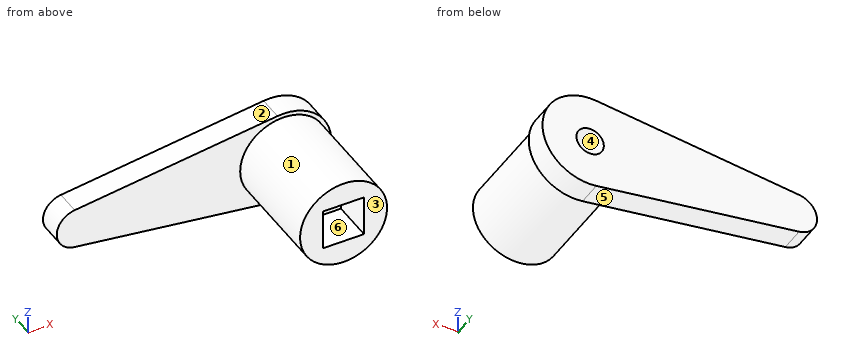
Solid Edge part; units mm, degrees
sketch "Sketch1" plane through (0, 0, 0) normal (0, 1, 0) x (-1, 0, 0)
  circle A0 centre (0, 0) radius 5.275
  circle A1 centre (0, 0) radius 1.66
extrude "Protrusion1" add sketch "Sketch1" along normal blind 8
sketch "Sketch2" plane through (0, 8, 0) normal (0, 1, 0) x (0, 0, 1)
  arc A0 (5.7252, -0.7565) -> (-5.7252, -0.7565) centre (0, 0) ccw
  line L0 (-2.4785, -25.3275) -> (-5.7252, -0.7565)
  arc A1 (-2.4785, -25.3275) -> (2.4785, -25.3275) centre (0, -25) ccw
  line L1 (2.4785, -25.3275) -> (5.7252, -0.7565)
  circle A2 centre (0, 0) radius 1.66
extrude "ExtrudedProtrusion_2" add sketch "Sketch2" along normal blind 3
sketch "Sketch3" plane through (0, 0, 0) normal (0, 1, 0) x (-1, 0, 0)
  line L0 (2.4732, 2.4732) -> (-2.4732, 2.4732)
  line L1 (-2.4732, 2.4732) -> (-2.4732, -2.4732)
  line L2 (-2.4732, -2.4732) -> (2.4732, -2.4732)
  line L3 (2.4732, -2.4732) -> (2.4732, 2.4732)
  circle A0 centre (0, 0) radius 5.275
extrude "ExtrudedProtrusion_5" add sketch "Sketch3" against normal blind 5
Source: CAD feature listing. Evaluate the final solid. Frame: model axes, mm. Face numbers are marked on the shaded views. A direction names the side the tool comes from. Give positions to 0.01 mm unless a question says otherwise; leave off trailing zeros. Loops run counter-clockwise (first coordinate to the right, second up) from the corner with the lowest first, then second, coordinate; pieces in that order, holes last. Notation, with made-up numbers: (68.25, 5) -> (103.25, 5) arc R18 cw to (103.25, 30) -> close; hole circle Ø5 at (89.5, 34.25). An arc over 180 degrees is marked (long way). Use a Markdown table: item, result. Add a question column.
1) Section query D-D, the plane y = 3.75. Return the cut outline in (x, z) (3 decimals).
2) Pull-direction query (X, two-part tool) for the marked faces 1, 2, 3 and 4; classes: +X half, -X half, draft (parallel to the pull), parting line (faces both ways), or undercut.
3) Reachability of the marked faces 5 and 6 from +Z, -Z, +X, -X, +Y, -Y: full face, straight path, thin tool, end or side. Return the list, or none.
4) Section query B-B, the plane z = 4.75. Return the cut outline in (x, y).
5) Line query: line 1 along Z through (x, y) = (0, 6) (3 decimals); line 2 along Y through (x, z) = (-13, -1.5); line 3 along Z through (x, y) = (-6, 9.5). Output: solid intervals per line, ascending. Write a range as [from, to].
6) Section query C-C, the plane x = 3. Return the cut outline in (y, z), then the cut area to 3 significant figures.
7) Section query A-A, the plane y = -3.25. Return the cut outline in (x, z) (3 decimals), then the cut area to 4 significant figures.
8) First-contact query: pin 1 (2.5 mm diameter, centred on x = -1, y = -2.5, fed in from -Z) (3 decimals); pin 2 (2.5 mm diameter, centred on x = 0, z = 0, fed in from +Y); pin 3 (2 mm diameter, centred on x = -23.5, y = 8, fed in from +Z); pin 4 (2.5 mm diameter, centred on y = -2, z = -0.5, fed in from -X) (3 decimals). Flat tips, straight axial feed; report the tip coordinate or a pass-through.
Numbers:
| question | item | result |
|---|---|---|
| 1 | outline | circle Ø10.55 at (0, 0); hole circle Ø3.32 at (0, 0) |
| 2 | face 1 | parting line |
| 2 | face 2 | -X half |
| 2 | face 3 | draft |
| 2 | face 4 | undercut |
| 3 | face 5 | -Z, -X, +Y, -Y |
| 3 | face 6 | -Y |
| 4 | outline | (-8.14, 8) -> (-2.29, 8) -> (-2.29, -5) -> (2.29, -5) -> (2.29, 8) -> (3.28, 8) -> (3.28, 11) -> (-8.14, 11) -> close |
| 5 | line 1 | z = [-5.275, -1.66], [1.66, 5.275] |
| 5 | line 2 | y = [8, 11] |
| 5 | line 3 | z = [-5.03, 5.03] |
| 6 | outline | (-5, -4.34) -> (8, -4.34) -> (8, -4.93) -> (11, -4.93) -> (11, 4.93) -> (8, 4.93) -> (8, 4.34) -> (-5, 4.34) -> close |
| 6 | area | 142 mm2 |
| 7 | outline | circle Ø10.55 at (0, 0); hole (-2.473, -2.473) -> (2.473, -2.473) -> (2.473, 2.473) -> (-2.473, 2.473) -> close |
| 7 | area | 62.95 mm2 |
| 8 | pin 1 | stops at z = -5.275 |
| 8 | pin 2 | passes through |
| 8 | pin 3 | stops at z = 2.85 |
| 8 | pin 4 | stops at x = -5.275 |
